Input: part model. Units: mm. Frame: model coordinates. A direction names the side the tool comes from. Give positions to 0.01 mm unless a question says otherwise; leave off trailing zeros. Order: outer loops, then holes, each group sorted by start corner. A loop starts at its lowest first (then second) coordinate and runs counter-clockwise, first axis right, second up. Notation, with made-up numbers: M -32.75,52.5 L -20.75,52.5 A20 ccw -20.75,65.5 Z; hole C 23,20 d8. An arc over 180 degrees is marked long. Use a Markdown table: item, result.
from build123d import *

# Parameters (mm, degrees)
SKETCH1_R                = 10
SKETCH1_R_2              = 5
EXTRUDE_THIN1_DEPTH      = 60
BOSS_EXTRUDE2_REACH      = 77.664
BOSS_EXTRUDE2_END_RADIUS = 10
SKETCH2_R                = 9
CUT_EXTRUDE1_REACH       = 77.664
CUT_EXTRUDE1_END_RADIUS  = 5
SKETCH3_R                = 5


with BuildPart() as part:
    # Sketch1 → Extrude-Thin1 (new body)
    with BuildSketch(Plane.XY):
        Circle(SKETCH1_R)
        Circle(SKETCH1_R_2, mode=Mode.SUBTRACT)
    extrude(amount=EXTRUDE_THIN1_DEPTH)

    # Boss-Extrude2: up to this cylinder (the profile starts outside it)
    boss_extrude2_end = Plane(origin=(0, 0, 30), z_dir=(0, 0, -1)) * Cylinder(BOSS_EXTRUDE2_END_RADIUS, 176.328, mode=Mode.PRIVATE)
    # Sketch2 → Boss-Extrude2 (add, up to the surface)
    with BuildSketch(Plane(origin=(35, 0, 0), x_dir=(0, 0, -1), z_dir=(1, 0, 0)), mode=Mode.PRIVATE) as boss_extrude2_sk1:
        with Locations((-30, 0)):
            Circle(SKETCH2_R)
    boss_extrude2_tool1 = extrude(boss_extrude2_sk1.sketch, amount=-BOSS_EXTRUDE2_REACH, mode=Mode.PRIVATE) - boss_extrude2_end
    add(boss_extrude2_tool1.solids().sort_by_distance((35, 0, 30))[0])

    # Cut-Extrude1: up to this cylinder (the profile starts outside it)
    cut_extrude1_end = Plane(origin=(0, 0, 29.948253), z_dir=(0, 0, -1)) * Cylinder(CUT_EXTRUDE1_END_RADIUS, 166.328, mode=Mode.PRIVATE)
    # Sketch3 → Cut-Extrude1 (cut, up to the surface)
    with BuildSketch(Plane(origin=(35, 0, 0), x_dir=(0, 0, -1), z_dir=(1, 0, 0)), mode=Mode.PRIVATE) as cut_extrude1_sk1:
        with Locations((-29.948253287, 0)):
            Circle(SKETCH3_R)
    cut_extrude1_tool1 = extrude(cut_extrude1_sk1.sketch, amount=-CUT_EXTRUDE1_REACH, mode=Mode.PRIVATE) - cut_extrude1_end
    add(cut_extrude1_tool1.solids().sort_by_distance((35, 0, 29.948253))[0], mode=Mode.SUBTRACT)


solid = part.part
1) First-contact query: pin 1 Ø1 at (y, z) = (-4.5, 26) entering from -X; pin 2 Ø8 at (x, z) = (10, 16.5) entering from -Y; pin 3 Ø5 at (x, y) = (23.5, -5) entering from +Z. Flat tips, straight axial feed; report the tip coordinate or a pass-through.
Response values:
| item | result |
|---|---|
| pin 1 | stops at x = -9.17 |
| pin 2 | stops at y = -8 |
| pin 3 | stops at z = 38.65 |
2) Cut plane D-D on y = 4. Return loops of the section in (x, z), and give its area (3 significant figures).
Response values:
| item | result |
|---|---|
| outline | M -9.17,0 L -3,0 L -3,60 L -9.17,60 Z; M 3,0 L 9.17,0 L 9.17,21.94 L 35,21.94 L 35,26.95 L 3,26.95 Z; M 3,32.95 L 35,32.95 L 35,38.06 L 9.17,38.06 L 9.17,60 L 3,60 Z |
| area | 964 mm² |
3) Mould query, pull axis Y, two halves, no side actions, for faces 3 (the face through (17.745, 0.22, 34.943)), 4 (the face through (-10, 0, 30)), 5 (the face through (-5, -2, 60)), 6 (the face through (-5, 0, 30)). Classes: released by +Y, released by -Y, zero draft, split by the parting line, or undercut.
Response values:
| item | result |
|---|---|
| face 3 | undercut |
| face 4 | split by the parting line |
| face 5 | zero draft |
| face 6 | undercut |
4) Cut plane B-B on z = 50. Return loops of the section in (x, y), and give its area (3 significant figures).
Response values:
| item | result |
|---|---|
| outline | C 0,0 d20; hole C 0,0 d10 |
| area | 236 mm² |
5) Reachability of faces 1 (the face through (35, -4, 26)), 2 (the face through (19.894, -3.447, 21.686)) from +Z, -Z, +X, -X, +Y, -Y: full face, straight path, thin tool, end or side. Return the list, or none.
Response values:
| item | result |
|---|---|
| face 1 | +Z, -Z, +X, +Y, -Y |
| face 2 | +X |
6) Cut plane C-C on x = 6. Return loops of the section in (y, z), and give its area (3 significant figures).
Response values:
| item | result |
|---|---|
| outline | M -8,0 L 8,0 L 8,25.88 A9 ccw 8,34.12 L 8,60 L -8,60 L -8,34.12 A9 ccw -8,25.88 Z; hole C 0,29.95 d10 |
| area | 893 mm² |
7) Cut plane A-A on y = 0. Return loops of the section in (x, z), and give its area (3 significant figures).
Response values:
| item | result |
|---|---|
| outline | M -10,0 L -5,0 L -5,60 L -10,60 Z; M 5,0 L 10,0 L 10,21 L 35,21 L 35,24.95 L 5,24.95 Z; M 5,34.95 L 35,34.95 L 35,39 L 10,39 L 10,60 L 5,60 Z |
| area | 750 mm² |
8) Material intervals for line 1 (Y direction, x = 0, z = 28.5); line 2 (X direction, y = 0.5, z = 55); line 3 (Y direction, x = -2, z = 19.5), sorted ascending. Write a range as from..to.
Response values:
| item | result |
|---|---|
| line 1 | y = -10..-5, 5..10 |
| line 2 | x = -9.99..-4.97, 4.97..9.99 |
| line 3 | y = -9.8..-4.58, 4.58..9.8 |
